from build123d import *

# Parameters (mm, degrees)
SKETCH_1_W      = 20
SKETCH_1_H      = 4.5
EXTRUDE_1_DEPTH = 12
FILLET_1_R      = 2
CHAMFER_1_SIZE  = 1


with BuildPart() as part:
    # 草圖1 → 旋轉1 (revolve)
    with BuildSketch(Plane.XY, mode=Mode.PRIVATE) as revolve_1_sk:
        with Locations((10, 2.25)):
            Rectangle(SKETCH_1_W, SKETCH_1_H)
    revolve(revolve_1_sk.sketch.rotate(Axis((0, 0, 0), (1, 0, 0)), 90), axis=Axis((0, 0, 0), (1, 0, 0)))

    # 草圖2 → 填料-伸長1 (add)
    with BuildSketch(Plane.ZY):
        Polygon((1.712942348, 6.713108707), (-4.957251505, 4.840005942), (-6.670193853, -1.873102765), (-1.712942348, -6.713108707), (4.957251505, -4.840005942), (6.670193853, 1.873102765), align=None)
    extrude(amount=EXTRUDE_1_DEPTH)

    # 圓角1
    fillet_1_edges = [part.edges().sort_by_distance(p)[0] for p in [
        (-12, 4.293105736, 4.1915681),
        (-12, 5.776557325, -1.622154578),
        (-12, 1.483451589, -5.813722679),
        (-12, -4.293105736, -4.1915681),
        (-12, -5.776557325, 1.622154578),
        (-12, -1.483451589, 5.813722679),
    ]]
    fillet(fillet_1_edges, radius=FILLET_1_R)

    # 導角1
    chamfer_1_edges = [part.edges().sort_by_distance(p)[0] for p in [
        (20, 0, -4.5),
        (0, 0, -4.5),
    ]]
    chamfer(chamfer_1_edges, length=CHAMFER_1_SIZE)


solid = part.part
Could you check a few things on this model? Use its own coordinates, in mm. A direction names the side the tool comes from. Round coordinates to 2 decimals unless told otherwise and drop trailing zeros. Write each loop counter-clockwise with the first axis right and the second up, starting at its lowest first coordinate (ties: lowest second). Pieces come first, ordered by that corner, then holes. Notation, with made-up numbers: (-18.75, -1.5) - (29.25, -1.5) arc R25 ccw to (29.25, 15.5) - close; hole circle Ø3 at (75, 65). An arc over 180 degrees is marked (long way). Put each result on its own line as item: value. Start each with the question number.
(1) I need wall thicknesses on probe 1 along Z at (x, y) = (-4, 0.5); probe 2 along Z at (x, y) = (4.5, 2.75); probe 3 along Y at (x, z) = (4.5, -0.5). Which ranges of each line are inside material? Lowest first, please.
(2) I want a section at A-A, the plane x = -3.5. Please give me the cut outline in (y, z), plus the area to 3 significant figures.
(3) For faces 1 (the flat face through (-4.93, 1.53, -5.8)), 2 (the cylindrical face through (10.13, -3.04, -3.32)), which set-ups out of +Z, -Z, +X, -X, +Y, -Y let a thin tool reach every point of the face, with its end or its side?
(4) Will these pins go through, and if not, where does the flat tip stop? pin 1 (5 mm diameter, centred on x = -7, y = 5, fed in from -Z); pin 2 (2 mm diameter, centred on x = -2.5, y = 0.5, fed in from +Z) (3 decimals); pin 3 (1 mm diameter, centred on x = -1.5, y = 0, fed in from +Z); pin 4 (6 mm diameter, centred on y = -2, z = 4.5, fed in from +X).
(5) I want a section at B-B, the plane x = 2.5. Please give me the cut outline in (y, z).
Here are the results:
1. probe 1: z = -6.06 to 6.32
1. probe 2: z = -3.56 to 3.56
1. probe 3: y = -4.47 to 4.47
2. outline: (-6.71, -1.71) - (-1.87, -6.67) - (4.84, -4.96) - (6.71, 1.71) - (1.87, 6.67) - (-4.84, 4.96) - close
2. area: 125 mm^2
3. face 1: -Z, +X, -X, +Y
3. face 2: +X
4. pin 1: stops at z = -5.55
4. pin 2: stops at z = 6.575
4. pin 3: stops at z = 6.32
4. pin 4: stops at x = 20
5. outline: circle Ø9 at (0, 0)
